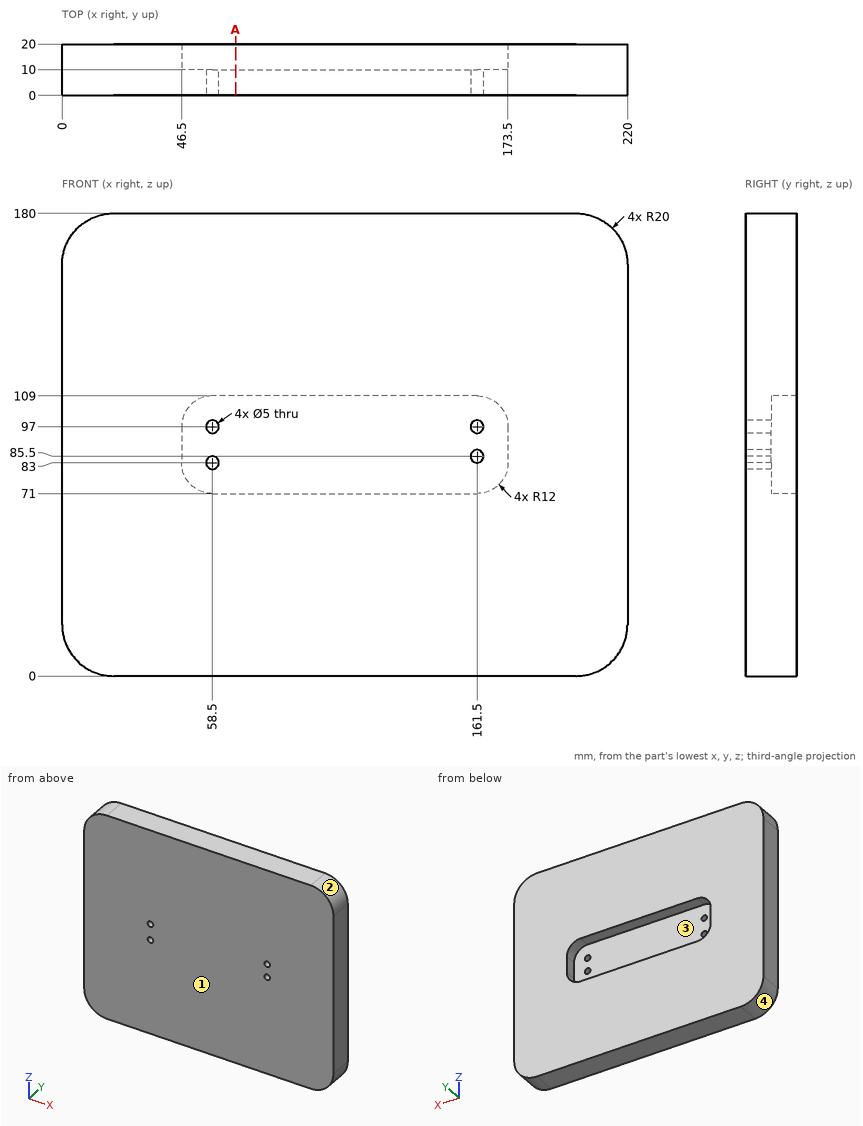
Print and shaded views of the part. All mm, measured from the part's lowest x, y and z. Round coordinates to 2 decimals unless told otherwise and drop trailing zeros. Loops run counter-clockwise (first coordinate to the right, second up) from the corner with the lowest first, then second, coordinate; pieces in that order, holes last. Notation, with made-up numbers: (-13.5, 33) -> (28.5, 33) arc R31 ccw to (28.5, 64) -> close; hole circle Ø8 at (88.5, 22). An arc over 180 degrees is marked (long way). Use CSV: the item, a comma, the result in double quotes. Start each with the question number.
1) Wall check: L1, parallel to Z at x = 58.5, y = 4.5; L2, parallel to Z at x = 161.5, y = 3.75; L3, parallel to Z at x = 157.5, y = 12. Give the ranges that are in metal, low to high. Write a range as [from, to].
2) Cut at A-A, the plane x = 67.5. Write the cut outline in (y, z).
3) Drop flat-ended pins along their axis: P1, Ø5, axis at y = 14.5, z = 89, coming from the -X side; P2, Ø8, axis at x = 161.5, z = 85.5, coming from the +Y side. Give the stop position or say it passes through.
4) Pull direction Z, two halves, no side cores. Call the marked faces 1, 2, 3 and 4: +Z half, -Z half, draft (parallel to the pull), parting line (faces both ways), or undercut.
Determined:
1,L1,"z = [0, 80.5], [85.5, 94.5], [99.5, 180]"
1,L2,"z = [0, 83], [88, 94.5], [99.5, 180]"
1,L3,"z = [0, 71], [109, 180]"
2,outline,"(0, 0) -> (20, 0) -> (20, 71) -> (10, 71) -> (10, 109) -> (20, 109) -> (20, 180) -> (0, 180) -> close"
3,P1,"stops at x = 0"
3,P2,"stops at y = 10"
4,face 1,"draft"
4,face 2,"+Z half"
4,face 3,"undercut"
4,face 4,"-Z half"
